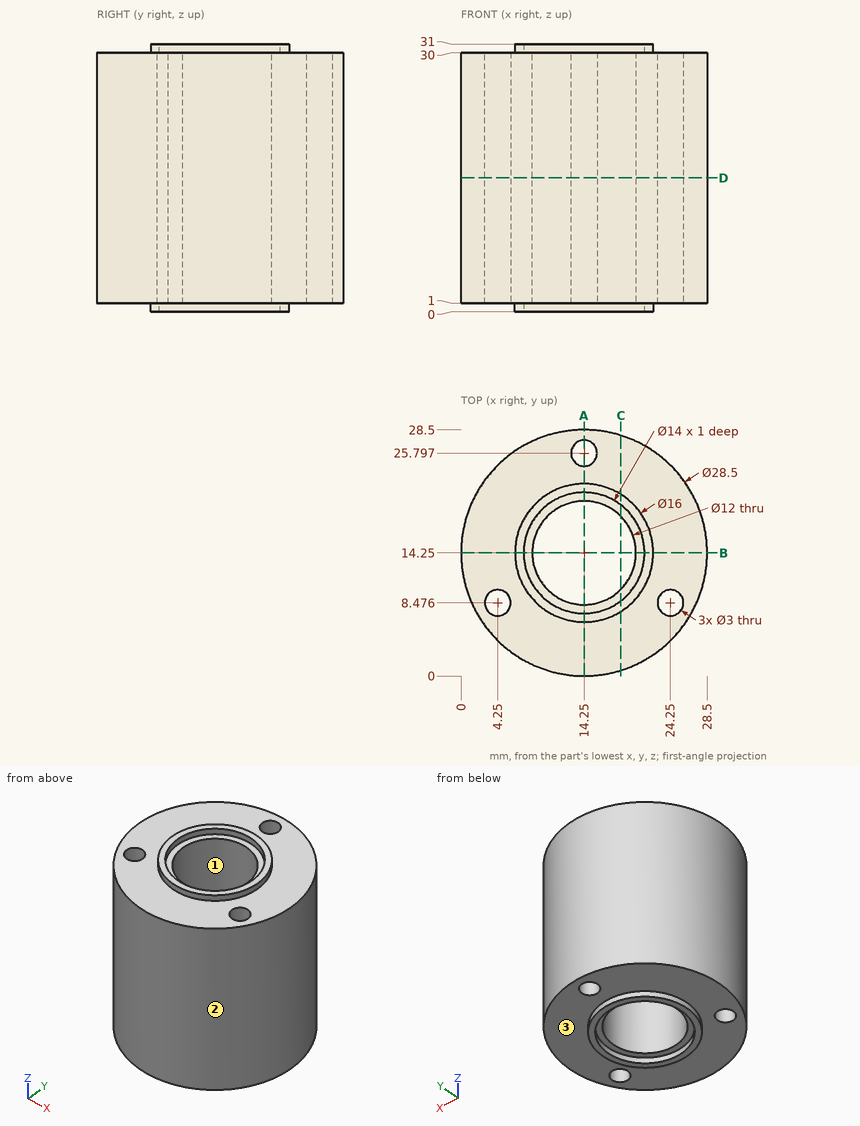
Answer from the drawing. Dimensions are ordinates in mm from the lowest x, y and z of the part. Coordinates: 2 decimals unless noted, no trailing zeros. Write each loop counter-clockwise with the first axis right and the second up, starting at its lowest first coordinate (ties: lowest second). Pieces come first, ordered by that corner, then holes. Notation, with made-up numbers: (39.25, 87.5) - (66.25, 87.5) arc R27 ccw to (66.25, 120.5) - close; hole circle Ø3 at (66, 53.5). An arc over 180 degrees is marked (long way). Return JSON: item names as keys, results as strings. Group by question number.
Q1. Flat-ended cylindrical pins translate along their axes: pin 1 Ø5 at (y, z) = (4, 25) entering from -X; pin 2 Ø6 at (x, z) = (23, 3) entering from -Y; pin 3 Ø3 at (x, z) = (7.5, 14) entering from -Y. Find the tip coordinate at first contact, or state that the pin passes through.
Q2. The part is cut by section B-B on y = 14.25. Write down the section's boundary in (x, z).
Q3. The part is cut by section C-C on x = 18.5. Write down the section's boundary in (y, z) (1 decimal), and give its area (3 significant figures).
Q4. The part is cut by section D-D on z = 15.5. Write down the section's boundary in (x, y).
Q5. For a pull along Y with two mould halves and no side action, classify the marked faces 1, 2 and 3 as +Y half, -Y half, draft (parallel to the pull), parting line (faces both ways), or undercut.
Q6. Find the intervals of material crossed by line 1 along Y through (x, z) = (13, 21.5) (1 decimal); line 2 along Z through (x, y) = (22.25, 24.5); line 3 along X through (y, z) = (11.5, 5), in increasing order. Write a range as [from, to].
Q7. The part is cut by section A-A on x = 14.25. Write down the section's boundary in (y, z).
Evaluation:
{
 "1": {"pin 1": "stops at x = 2.29", "pin 2": "stops at y = 1.21", "pin 3": "stops at y = 1"},
 "2": {"outline": "(0, 1) - (6.25, 1) - (6.25, 0) - (7.25, 0) - (7.25, 1) - (8.25, 1) - (8.25, 30) - (7.25, 30) - (7.25, 31) - (6.25, 31) - (6.25, 30) - (0, 30) - close; (20.25, 1) - (21.25, 1) - (21.25, 0) - (22.25, 0) - (22.25, 1) - (28.5, 1) - (28.5, 30) - (22.25, 30) - (22.25, 31) - (21.25, 31) - (21.25, 30) - (20.25, 30) - close"},
 "3": {"outline": "(0.6, 1) - (7.5, 1) - (7.5, 0) - (8.7, 0) - (8.7, 1) - (10, 1) - (10, 30) - (8.7, 30) - (8.7, 31) - (7.5, 31) - (7.5, 30) - (0.6, 30) - close; (18.5, 1) - (19.8, 1) - (19.8, 0) - (21, 0) - (21, 1) - (27.9, 1) - (27.9, 30) - (21, 30) - (21, 31) - (19.8, 31) - (19.8, 30) - (18.5, 30) - close", "area": "548 mm2"},
 "4": {"outline": "circle Ø28.5 at (14.25, 14.25); hole circle Ø3 at (4.25, 8.48); hole circle Ø12 at (14.25, 14.25); hole circle Ø3 at (14.25, 25.8); hole circle Ø3 at (24.25, 8.48)"},
 "5": {"face 1": "undercut", "face 2": "parting line", "face 3": "draft"},
 "6": {"line 1": "y = [0.1, 8.4], [20.1, 25], [26.6, 28.4]", "line 2": "z = [1, 30]", "line 3": "x = [0.27, 8.92], [19.58, 28.23]"},
 "7": {"outline": "(0, 1) - (6.25, 1) - (6.25, 0) - (7.25, 0) - (7.25, 1) - (8.25, 1) - (8.25, 30) - (7.25, 30) - (7.25, 31) - (6.25, 31) - (6.25, 30) - (0, 30) - close; (20.25, 1) - (21.25, 1) - (21.25, 0) - (22.25, 0) - (22.25, 1) - (24.3, 1) - (24.3, 30) - (22.25, 30) - (22.25, 31) - (21.25, 31) - (21.25, 30) - (20.25, 30) - close; (27.3, 1) - (28.5, 1) - (28.5, 30) - (27.3, 30) - close"}
}
